Solid Edge part; units mm, degrees
sketch "Sketch1" plane through (0, 0, 0) normal (0, 0, 1) x (1, 0, 0)
  circle A0 centre (0, 0) radius 20
  circle A1 centre (0, 0) radius 2
extrude "ExtrudedProtrusion_1" add sketch "Sketch1" along normal blind 20
sketch "Sketch2" plane through (0, 0, 20) normal (0, 0, 1) x (1, 0, 0)
  line L0 (-0.7616, -9.485) -> (4.95, -19.3778)
  line L1 (-12.02, -15.985) -> (-0.7616, -9.485)
  arc A0 (4.95, -19.3778) -> (-12.02, -15.985) centre (0, 0) cw
  line L2 (-0.7616, 9.485) -> (4.95, 19.3778)
  line L3 (-12.02, 15.985) -> (-0.7616, 9.485)
  arc A1 (4.95, 19.3778) -> (-12.02, 15.985) centre (0, 0) ccw
extrude "ExtrudedCutout_1" cut sketch "Sketch2" against normal blind 10
sketch "Sketch3" plane through (-6.3908, -12.735, 15) normal (0.5, -0.8660254, 0) x (0.8660254, 0.5, 0)
  circle A0 centre (0, 0) radius 2.5
extrude "ExtrudedCutout_2" cut sketch "Sketch3" against normal blind 10
mirror "Mirror1" about plane through (0, 0, 0) normal (0, -1, 0) of "ExtrudedCutout_2"
properties material "Aluminio"
Design review of the part built by this model. Coordinates are the model's own, in mm. A direction names the side the tool comes from. Give positions to 0.01 mm unless a question says otherwise; leave off trailing zeros. Loops run counter-clockwise (first coordinate to the right, second up) from the corner with the lowest first, then second, coordinate; pieces in that order, holes last. Notation, with made-up numbers: (1.25, -37.5) -> (16.25, -37.5) arc R8 cw to (16.25, -26.5) -> close; hole circle Ø3 at (20.5, 52). An arc over 180 degrees is marked (long way). One line per question, with ' | ' between items. Start each with the question number.
(1) For faces 4 (the face through (-7.721, 13.503, 17.292)), 5 (the face through (-11.36, -4.057, 14.965)), 6 (the face through (2.054, -14.362, 15.07)), list the 3-axis set-ups (+Z, -Z, +X, -X, +Y, -Y) from which the entire face can be reached by the end or side of a thin tool; tool diameter is ignored.
(2) We need section D-D (z = 6.25). State the section outline as (x, y) points, and give its area (3 significant figures).
(3) Draft analysis for pull direction X (two halves, no side actions). For faces 1 (the face through (18.475, 7.66, 9.86)), 2 (the face through (4, 0, 0)), 3 (the face through (-11.02, -9.71, 15.11)), state which applies: +X half, -X half, draft (parallel to the pull), parting line (faces both ways), or undercut.
(4) We need section C-C (x = -16). State the section outline as (y, z) points.
(5) We need section A-A (y = 0). State the section outline as (x, z) points.
(6) For line 1 (Y direction, x = -12, z = 15.25); line 2 (Y direction, x = 0, z = 8); line 3 (Z direction, x = -1, y = -17.5), list the stretches that pass through material, from the lowest coordinate up.
(7) We need section B-B (x = 0). State the section outline as (y, z) points.
(8) Insertion check: P1, Ø1.5, axis at y = 14.5, z = 17.5, coming from the -X side; P2, Ø8, axis at y = 6, z = 8.5, coming from the -X side; P3, Ø3, axis at x = -4.5, y = 14, coming from the +Z side. Each pin has a flat end and moves straight along its axis. Give the tip position at first contact, or say it passes through.
The answers:
1) face 4: +Z, +Y | face 5: none | face 6: +Z, -Y
2) outline: circle Ø40 at (0, 0); hole circle Ø4 at (0, 0) | area: 1,240 mm^2
3) face 1: parting line | face 2: draft | face 3: undercut
4) outline: (-12, 0) -> (12, 0) -> (12, 20) -> (-12, 20) -> close
5) outline: (-20, 0) -> (-2, 0) -> (-2, 20) -> (-20, 20) -> close; (2, 0) -> (20, 0) -> (20, 20) -> (2, 20) -> close
6) line 1: y = -15.97 to -7.99, -4.43 to 4.43, 7.99 to 15.97 | line 2: y = -20 to -2, 2 to 20 | line 3: z = 0 to 10
7) outline: (-20, 0) -> (-2, 0) -> (-2, 20) -> (-10.8, 20) -> (-10.8, 10) -> (-20, 10) -> close; (2, 0) -> (20, 0) -> (20, 10) -> (10.8, 10) -> (10.8, 20) -> (2, 20) -> close
8) P1: stops at x = -14.52 | P2: stops at x = -19.9 | P3: stops at z = 10
